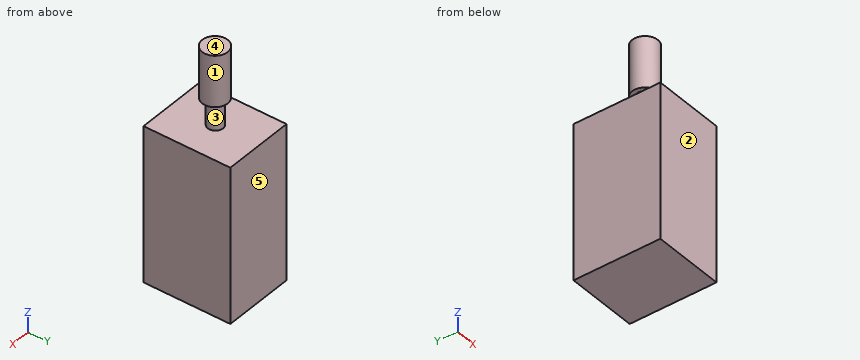
```python
from build123d import *

# Parameters (mm, degrees)
SKETCH1_W           = 30.4
SKETCH1_H           = 17
BOSS_EXTRUDE1_DEPTH = 14
SKETCH2_R           = 1.5
BOSS_EXTRUDE2_DEPTH = 5.4
SKETCH3_R           = 2.5
BOSS_EXTRUDE3_DEPTH = 10


with BuildPart() as part:
    # Sketch1 → Boss-Extrude1 (new body)
    with BuildSketch(Plane(origin=(0, 0, 0), x_dir=(0, 0, -1), z_dir=(1, 0, 0))):
        Rectangle(SKETCH1_W, SKETCH1_H)
    extrude(amount=BOSS_EXTRUDE1_DEPTH)

    # Sketch2 → Boss-Extrude2 (add)
    with BuildSketch(Plane.XY.offset(15.2)):
        with Locations(Location((6.88711981, 0, 0), (0, 0, 180))):
            Circle(SKETCH2_R)
    extrude(amount=BOSS_EXTRUDE2_DEPTH)

    # Sketch3 → Boss-Extrude3 (add)
    with BuildSketch(Plane.XY.offset(20.6)):
        with Locations((7, 0)):
            Circle(SKETCH3_R)
    extrude(amount=BOSS_EXTRUDE3_DEPTH)


solid = part.part
```
Here's how the part is built. I have some questions about the finished solid (model axes, mm). Face numbers are marked on the shaded views. A direction names the side the tool comes from. Coordinates: 2 decimals unless noted, no trailing zeros. Order: outer loops, then holes, each group sorted by start corner. A loop starts at its lowest first (then second) coordinate and runs counter-clockwise, first axis right, second up.
1) Imagine slicing it at D-D on x = 7. List the corners of the cut face in (y, z) for me.
2) Which directions (+Z, -Z, +X, -X, +Y, -Y) give clear straight access to the entire face, cutting with the end or side of a thin tool? Please do the marked faces 1 and 2.
3) I need wall thicknesses on line 1 (Z direction, x = 5.5, y = 1.75); line 2 (Z direction, x = 5.25, y = -3); line 3 (Y direction, x = 7, z = 22). Which ranges of each line are inside material? Lowest first, please.
4) Imagine slicing it at B-B on y = 0. List the corners of the cut face in (x, z) for me.
5) Imagine slicing it at A-A on y = -2. List the corners of the cut face in (x, z) for me, and give its area (3 significant figures).
6) Imagine slicing it at C-C on z = 18.5. List the corners of the cut face in (x, y) for me, and give its area (3 significant figures).
7) We'd pull the mould along Z, two halves only. Please class the marked faces 3, 4 and 5: +Z half, -Z half, draft (parallel to the pull), parting line (faces both ways), or undercut.
8) Will this pin go through, and if not, where does the flat tip stop? pin 1 (3 mm diameter, centred on x = 3.5, z = 21.5, fed in from +Y).
Response values:
1. outline: (-8.5, -15.2) - (8.5, -15.2) - (8.5, 15.2) - (1.5, 15.2) - (1.5, 20.6) - (2.5, 20.6) - (2.5, 30.6) - (-2.5, 30.6) - (-2.5, 20.6) - (-1.5, 20.6) - (-1.5, 15.2) - (-8.5, 15.2) - close
2. face 1: +Z
2. face 2: +Z, -Z, +X, -X, -Y
3. line 1: z = -15.2 to 15.2, 20.6 to 30.6
3. line 2: z = -15.2 to 15.2
3. line 3: y = -2.5 to 2.5
4. outline: (0, -15.2) - (14, -15.2) - (14, 15.2) - (8.39, 15.2) - (8.39, 20.6) - (9.5, 20.6) - (9.5, 30.6) - (4.5, 30.6) - (4.5, 20.6) - (5.39, 20.6) - (5.39, 15.2) - (0, 15.2) - close
5. outline: (0, -15.2) - (14, -15.2) - (14, 15.2) - (0, 15.2) - close; (5.5, 20.6) - (8.5, 20.6) - (8.5, 30.6) - (5.5, 30.6) - close
5. area: 456 mm2
6. outline: circle Ø3 at (6.89, 0)
6. area: 7.07 mm2
7. face 3: undercut
7. face 4: +Z half
7. face 5: draft
8. pin 1: stops at y = 1.5
